from build123d import *

# Parameters (mm, degrees)
SKETCH1_W           = 760
SKETCH1_H           = 98.2
SKETCH1_W_2         = 700
SKETCH1_H_2         = 38.2
BOSS_EXTRUDE3_DEPTH = 40.64
SKETCH2_W           = 700
SKETCH2_H           = 38.2
BOSS_EXTRUDE4_DEPTH = 0.254
SKETCH3_W           = 67.5
SKETCH3_H           = 43.5
CUT_EXTRUDE1_DEPTH  = 40.386
SKETCH6_R           = 18
SKETCH6_R_2         = 12.8397
BOSS_EXTRUDE5_DEPTH = 15
SKETCH7_W           = 38.1
SKETCH7_H           = 44.37
BOSS_EXTRUDE6_DEPTH = 20


with BuildPart() as part:
    # Sketch1 → Boss-Extrude3 (new body)
    with BuildSketch(Plane(origin=(0, 0, 0), x_dir=(1, 0, 0), z_dir=(0, 1, 0))):
        Rectangle(SKETCH1_W, SKETCH1_H)
        Rectangle(SKETCH1_W_2, SKETCH1_H_2, mode=Mode.SUBTRACT)
    extrude(amount=BOSS_EXTRUDE3_DEPTH)

    # Sketch2 → Boss-Extrude4 (add)
    with BuildSketch(Plane.XZ):
        Rectangle(SKETCH2_W, SKETCH2_H)
    extrude(amount=-BOSS_EXTRUDE4_DEPTH)

    # Sketch3 → Cut-Extrude1 (cut)
    with BuildSketch(Plane(origin=(0, 40.64, 0), x_dir=(1, 0, 0), z_dir=(0, 1, 0))):
        with Locations((316.25, 0)):
            Rectangle(SKETCH3_W, SKETCH3_H)
    extrude(amount=-CUT_EXTRUDE1_DEPTH, mode=Mode.SUBTRACT)

    # Sketch6 → Boss-Extrude5 (add)
    with BuildSketch(Plane(origin=(-350, 0, 0), x_dir=(0, 0, -1), z_dir=(1, 0, 0))):
        with Locations((0, 20.32)):
            Circle(SKETCH6_R)
        with Locations((0, 20.32)):
            Circle(SKETCH6_R_2, mode=Mode.SUBTRACT)
    extrude(amount=BOSS_EXTRUDE5_DEPTH)

    # Sketch7 → Boss-Extrude6 (add)
    with BuildSketch(Plane.XZ):
        Rectangle(SKETCH7_W, SKETCH7_H)
    extrude(amount=BOSS_EXTRUDE6_DEPTH)


solid = part.part
Model file for the job. Use its own axes, mm. A direction names the side the tool comes from. Give positions to 0.01 mm unless a question says otherwise; leave off trailing zeros. Order: outer loops, then holes, each group sorted by start corner. A loop starts at its lowest first (then second) coordinate and runs counter-clockwise, first axis right, second up. Notation, with made-up numbers: (-38, 24.25) - (13, 24.25) arc R24 cw to (13, 46.25) - close; hole circle Ø3 at (2, 67). An arc over 180 degrees is marked (long way). Write item = value, one per line. Start each with the question number.
1. Two-plate mould, pull along Z, no slides. Class faces 1 (the flat face through (-380, 20, 1)), 2 (the flat face through (-5, 20, -49.1)), 3 (the flat face through (-335, 24.6, 12.3)), 4 (the flat face through (-5, 20, 49.1)): pulls with the +Z half, pulls with the -Z half, needs draft (parallel to the pull), parting line crosses it, or undercut.
2. Cut at A-A, the plane y = 20.32. List the corners of the cut face in (x, z), and give its area (3 significant figures).
3. Cut at D-D, the plane z = -41. List the corners of the cut face in (x, y), and give its area (3 significant figures).
4. Drop flat-ended pins along their axis: P1, Ø8, axis at y = -7, z = -39, coming from the +X side; P2, Ø10, axis at x = 280.5, z = -20, coming from the -Y side; P3, Ø16, axis at y = -9, z = 1.5, coming from the +X side. Give the stop position or say it passes through.
5. Probe line 1 along Y through (x, z) = (-338.25, 0); line 2 along Z through (x, y) = (-339, 20); line 3 along X through (y, z) = (15.5, 14). List the from-to ranges inside material, lowest first.
6. Cut at C-C, the plane x = -220. List the corners of the cut face in (y, z).
7. Which spindle directions (+Z, -Z, +X, -X, +Y, -Y) get a long thin tool onto all of the face, cutting with end or side? Do faces 5 (the cylindrical face through (-342.6, 33.05, 1.67)), 6 (the flat face through (-38, 20, 19.1)), 7 (the flat face through (19.05, -10, 0)), 8 (the flat face through (-19.05, -10, 0)), 9 (the flat face through (0, -10, -22.185)). Say none if no direction does.
8. Cut at B-B, the plane z = 0. List the corners of the cut face in (x, y).
Taken from the geometry:
q1.face_1 = needs draft
q1.face_2 = pulls with the -Z half
q1.face_3 = undercut
q1.face_4 = pulls with the +Z half
q2.outline = (-380, -49.1) - (380, -49.1) - (380, 49.1) - (-380, 49.1) - close; hole (-350, -19.1) - (282.5, -19.1) - (282.5, -21.75) - (350, -21.75) - (350, 21.75) - (282.5, 21.75) - (282.5, 19.1) - (-350, 19.1) - (-350, 18) - (-335, 18) - (-335, 12.84) - (-350, 12.84) - (-350, -12.84) - (-335, -12.84) - (-335, -18) - (-350, -18) - close
q2.area = 47,700 mm²
q3.outline = (-380, 0) - (380, 0) - (380, 40.64) - (-380, 40.64) - close
q3.area = 30,900 mm²
q4.P1 = through
q4.P2 = 0
q4.P3 = 19.05
q5.line_1 = 0 to 0.25, 2.32 to 7.48, 33.16 to 38.32
q5.line_2 = -49.1 to -19.1, -18 to -12.84, 12.84 to 18, 19.1 to 49.1
q5.line_3 = -380 to -335, 350 to 380
q6.outline = (0, -49.1) - (40.64, -49.1) - (40.64, -19.1) - (0.25, -19.1) - (0.25, 19.1) - (40.64, 19.1) - (40.64, 49.1) - (0, 49.1) - close
q7.face_5 = none
q7.face_6 = +Y
q7.face_7 = +Z, -Z, +X, -Y
q7.face_8 = +Z, -Z, -X, -Y
q7.face_9 = -Z, +X, -X, -Y
q8.outline = (-380, 0) - (-19.05, 0) - (-19.05, -20) - (19.05, -20) - (19.05, 0) - (380, 0) - (380, 40.64) - (350, 40.64) - (350, 0.25) - (-350, 0.25) - (-350, 2.32) - (-335, 2.32) - (-335, 7.48) - (-350, 7.48) - (-350, 33.16) - (-335, 33.16) - (-335, 38.32) - (-350, 38.32) - (-350, 40.64) - (-380, 40.64) - close
